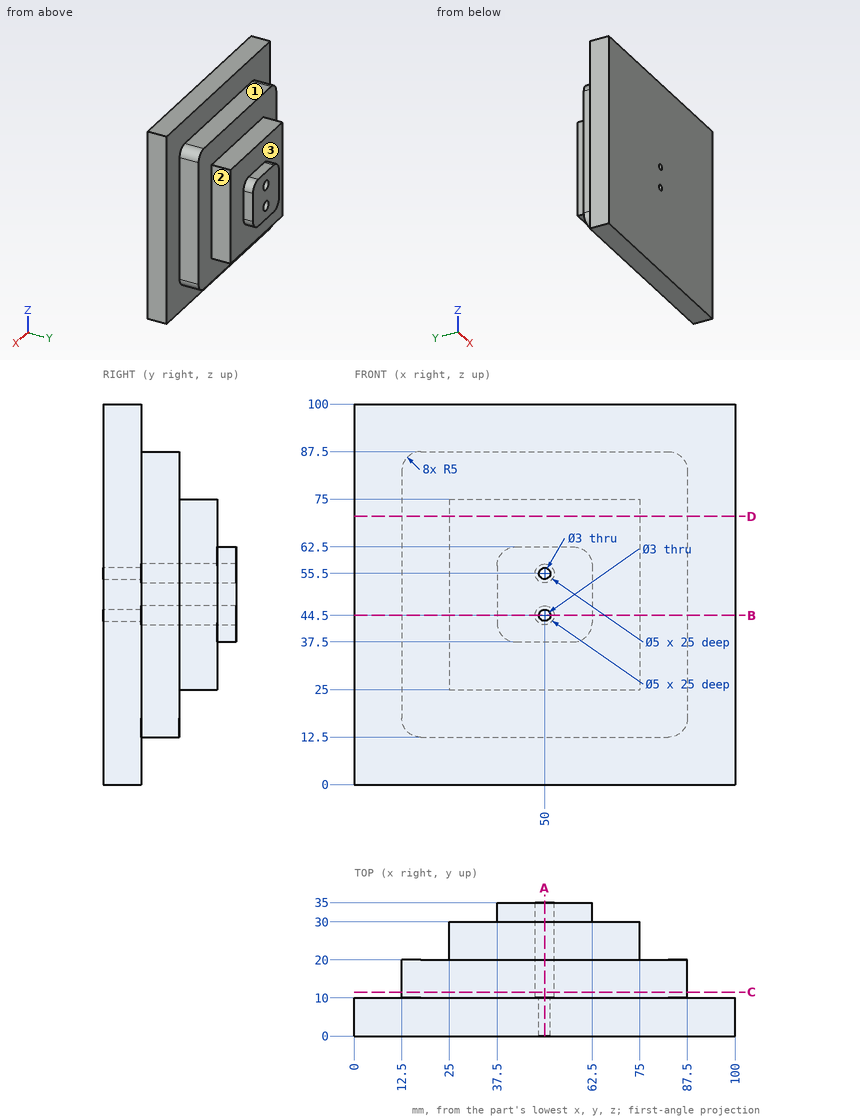
Geometry: see drawing. Coordinates: mm, zero at the bounding-box minimum. A direction names the side the tool comes from. Coordinates: 2 decimals unless noted, no trailing zeros. Loops run counter-clockwise (first coordinate to the right, second up) from the corner with the lowest first, then second, coordinate; pieces in that order, holes last. Notation, with made-up numbers: (15, 21.5) - (72, 21.5) arc R13 ccw to (72, 27.5) - close; hole circle Ø2 at (39.5, 72). An arc over 180 degrees is marked (long way). Answer in a Markdown table with one row per item.
(1) Cut plane D-D on z = 70.5. Output: boundary loops of the cut face in (x, y), plus the area to 3 significant figures.
Model answer:
| item | result |
|---|---|
| outline | (0, 0) - (100, 0) - (100, 10) - (87.5, 10) - (87.5, 20) - (75, 20) - (75, 30) - (25, 30) - (25, 20) - (12.5, 20) - (12.5, 10) - (0, 10) - close |
| area | 2,250 mm² |
(2) Cut plane C-C on y = 11.5. Output: boundary loops of the cut face in (x, z).
Model answer:
| item | result |
|---|---|
| outline | (12.5, 17.5) arc R5 ccw to (17.5, 12.5) - (82.5, 12.5) arc R5 ccw to (87.5, 17.5) - (87.5, 82.5) arc R5 ccw to (82.5, 87.5) - (17.5, 87.5) arc R5 ccw to (12.5, 82.5) - close; hole circle Ø5 at (50, 44.5); hole circle Ø5 at (50, 55.5) |
(3) Cut plane A-A on x = 50. Count the separate pieces of the cut face and the enclosed holes in it, plus the area to 4 significant figures.
Model answer:
| item | result |
|---|---|
| separate pieces | 3 |
| enclosed holes | 0 |
| area | 2,065 mm² |
(4) Cut plane B-B on z = 44.5. Output: boundary loops of the cut face in (x, y).
Model answer:
| item | result |
|---|---|
| outline | (0, 0) - (48.5, 0) - (48.5, 10) - (47.5, 10) - (47.5, 35) - (37.5, 35) - (37.5, 30) - (25, 30) - (25, 20) - (12.5, 20) - (12.5, 10) - (0, 10) - close; (51.5, 0) - (100, 0) - (100, 10) - (87.5, 10) - (87.5, 20) - (75, 20) - (75, 30) - (62.5, 30) - (62.5, 35) - (52.5, 35) - (52.5, 10) - (51.5, 10) - close |
(5) Set-up query: the marked faces 1, 2 and 3. Return all of +Z, -Z, +X, -X, +Y, -Y with unobstructed straight access to the full face (end or side cutting, diameter ignored); none if empty.
Model answer:
| item | result |
|---|---|
| face 1 | +Z, +X, -X, +Y |
| face 2 | +Z, -Z, +X, +Y |
| face 3 | +Y |
(6) Pin query (flat end, axial travel): P1, Ø5, axis at y = 13.5, z = 60.5, coming from the -X side; P2, Ø1.5, axis at x = 49, z = 44.5, coming from the +Y side; P3, Ø1, axis at y = 21, z = 70.5, coming from the -X side; P4, Ø1.8, axis at x = 50, z = 55.5, coming from the +Y side. Return the tip coordinate at first contact, or that it passes through.
Model answer:
| item | result |
|---|---|
| P1 | stops at x = 12.5 |
| P2 | stops at y = 10 |
| P3 | stops at x = 25 |
| P4 | passes through |
(7) Material intervals for L1, parallel to X at y = 21, z = 55.5; L2, parallel to Z at x = 37, y = 15.5; L3, parallel to Y at x = 81, z = 56, sorted ascending. Write a range as from..to.
Model answer:
| item | result |
|---|---|
| L1 | x = 25..47.5, 52.5..75 |
| L2 | z = 12.5..87.5 |
| L3 | y = 0..20 |
